Source: CAD feature listing. Evaluate the final solid. Frame: model axes, mm. Face numbers are marked on the shaded views. A direction names the side the tool comes from. Give positions to 0.01 mm unless a question says otherwise; leave off trailing zeros. Order: outer loops, then holes, each group sorted by start corner. A loop starts at its lowest first (then second) coordinate and runs counter-clockwise, first axis right, second up. Notation, with made-up numbers: (58.25, -10) - (80.25, -10) arc R12 ccw to (80.25, -5) - close; hole circle Ø7 at (32, -11). An arc over 180 degrees is marked (long way). Answer as CSV lines item,"result".
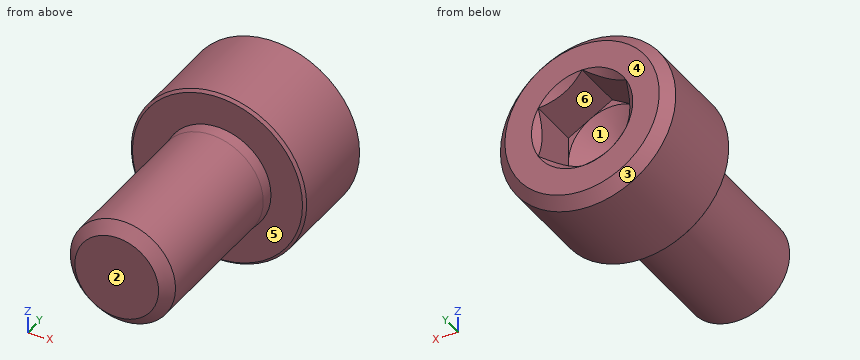
```python
from build123d import *

# Parameters (mm, degrees)
CUT_EXTRUDE1_DEPTH = 3


with BuildPart() as part:
    # Sketch1 → Revolve1 (revolve)
    with BuildSketch(Plane.XY):
        Polygon((0, 1.556624327), (2.5, 3), (2.5, 5.613248654), (2.886751346, 6), (4.4, 6), (5, 5.4), (5, 0.15), (4.85, 0), (3.05, 0), (3, -0.68), (3, -9.3865), (2.3865, -10), (0, -10), align=None)
    revolve(axis=Axis((0, -10, 0), (0, 1, 0)))

    # Sketch2 → Cut-Extrude1 (cut)
    with BuildSketch(Plane(origin=(0, 6, 0), x_dir=(1, 0, 0), z_dir=(0, 1, 0))):
        Polygon((-2.5, -1.443375673), (0, -2.886751346), (2.5, -1.443375673), (2.5, 1.443375673), (0, 2.886751346), (-2.5, 1.443375673), align=None)
    extrude(amount=-CUT_EXTRUDE1_DEPTH, mode=Mode.SUBTRACT)


solid = part.part
```
(1) Contact query for flat-ended pins moving along their axis: pin 1 (1.5 mm diameter, centred on y = -5, z = 2.5, fed in from +X); pin 2 (0.6 mm diameter, centred on x = 1.5, z = 1.5, fed in from +Y); pin 3 (1 mm diameter, centred on y = 3.5, z = 1.5, fed in from +X); pin 4 (1.4 mm diameter, centred on y = 4, z = -0.5, fed in from -X). Output: stop coordinate, or through.
Completed:
pin 1,"x = 2.44"
pin 2,"y = 2.95"
pin 3,"x = 4.9"
pin 4,"x = -5"
(2) Cut plane C-C (y = -0.25). Return loops of the section in (x, z), then the cut area to 3 significant figures.
Completed:
outline,"circle Ø6.06 at (0, 0)"
area,"28.9 mm²"
(3) Mould query, pull axis X, two halves, no side actions, for the marked faces 1, 2 and 3. Classes: released by +X, released by -X, zero draft, split by the parting line, or undercut.
Completed:
face 1,"undercut"
face 2,"zero draft"
face 3,"split by the parting line"
(4) Cut plane B-B (y = -3.25). Return loops of the section in (x, z).
Completed:
outline,"circle Ø6 at (0, 0)"
(5) Access query for the marked faces 4, 5 and 6. Directions: +Z, -Z, +X, -X, +Y, -Y. A direction counts if a zero-diameter tool reaches every point of the face in a straight line with its end or side. Return the directions, or none.
Completed:
face 4,"+Z, -Z, +X, -X, +Y"
face 5,"-Y"
face 6,"+Y"
(6) Cut plane A-A (y = 4.5). Return loops of the section in (x, z), then the cut area to 3 significant figures.
Completed:
outline,"circle Ø10 at (0, 0); hole (-2.5, -1.44) - (0, -2.89) - (2.5, -1.44) - (2.5, 1.44) - (0, 2.89) - (-2.5, 1.44) - close"
area,"56.9 mm²"
(7) Ray query, line 1 (Z direction, x = 4, y = 0.25); line 2 (Y direction, x = -3, z = 3); line 3 (Z direction, x = 0.5, y = 2.75). Return the intervals inside material, ascending. Write a range as from..to.
Completed:
line 1,"-3..3"
line 2,"0..6"
line 3,"-4.97..-2.01, 2.01..4.97"
